Could you check a few things on this model? Use its own coordinates, in mm. Face numbers are marked on the shaded views. Coordinates: 2 decimals unless noted, no trailing zeros. Order: outer loops, then holes, each group sorted by start corner. A loop starts at its lowest first (then second) coordinate and runs counter-clockwise, first axis right, second up. Notation, with made-up numbers: (16.5, 52) -> (38.5, 52) arc R33 ccw to (38.5, 88) -> close; hole circle Ø4 at (-21.75, 65). An arc over 180 degrees is marked (long way). Use a Markdown table: item, result. Add a question column.
1) If we section it at A-A (z = 0): Write out the boundary of the cut face in (x, y).
2) If I drill on L1, parallel to X at y = 41.4, z = 0; L2, parallel to Y at x = 40, z = -10; L3, parallel to Z at x = -78.5, y = -21, over which ranges is the centre line in solid material (lowest first)? Write a range as [from, to].
3) If we section it at D-D (x = -11.5): Write out the boundary of the cut face in (y, z), plus the area to 3 significant figures.
4) Will these pins go through, and if not, where does the flat tip stop? pin 1 Ø4 at (x, y) = (-32.5, 14) entering from -Z; pin 2 Ø6 at (x, z) = (51, -12.5) entering from -Y; pin 3 Ø9 at (x, z) = (-75, 0) entering from +Y; pin 4 Ø2 at (x, z) = (-42, -4) entering from +Y.
5) If we section it at B-B (y = 0): Write out the boundary of the cut face in (x, z), plus the area to 3 significant figures.
6) Thinking about a two-plate mould opening in Y: for the marked faces 1 and 2, which applies, +Y half, -Y half, draft (parallel to the pull), parting line (faces both ways), or undercut?
Solid Edge part; units mm, degrees
sketch "Sketch1" plane through (0, 0, 0) normal (1, 0, 0) x (0, 1, 0)
  circle A0 centre (0, 0) radius 42.5
extrude "Protrusion1" add sketch "Sketch1" along normal mid plane 200
sketch "Sketch2" plane through (0, 0, 0) normal (1, 0, 0) x (0, 1, 0)
  circle A0 centre (0, 0) radius 41
extrude "ExtrudedCutout_5" cut sketch "Sketch2" along normal mid plane 200
sketch "Sketch3" plane through (0, 0, 0) normal (0, -1, 0) x (1, 0, 0)
  circle A0 centre (75, 0) radius 4
extrude "ExtrudedCutout_9" cut sketch "Sketch3" along normal mid plane 90
sketch "Sketch4" plane through (0, 0, 0) normal (0, -1, 0) x (1, 0, 0)
  circle A0 centre (-75, 0) radius 4
extrude "ExtrudedProtrusion_6" cut sketch "Sketch4" along normal mid plane 90
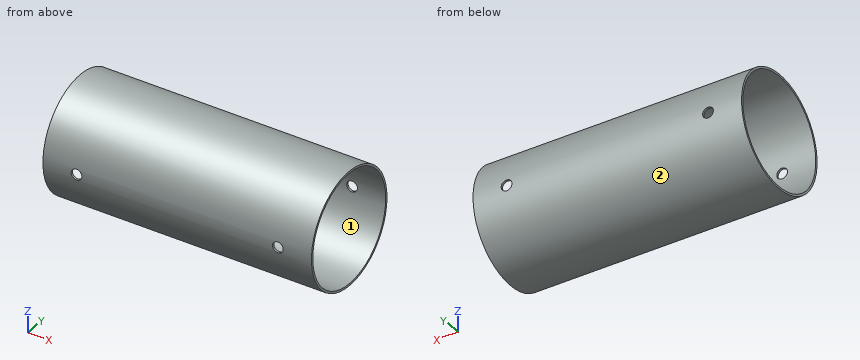
Answer sheet:
| question | item | result |
|---|---|---|
| 1 | outline | (-100, -42.5) -> (-79, -42.5) -> (-79, -41) -> (-100, -41) -> close; (-100, 41) -> (-79, 41) -> (-79, 42.5) -> (-100, 42.5) -> close; (-71, -42.5) -> (71, -42.5) -> (71, -41) -> (-71, -41) -> close; (-71, 41) -> (71, 41) -> (71, 42.5) -> (-71, 42.5) -> close; (79, -42.5) -> (100, -42.5) -> (100, -41) -> (79, -41) -> close; (79, 41) -> (100, 41) -> (100, 42.5) -> (79, 42.5) -> close |
| 2 | L1 | [-100, -79], [-71, 71], [79, 100] |
| 2 | L2 | [-41.31, -39.76], [39.76, 41.31] |
| 2 | L3 | [-36.95, -35.21], [35.21, 36.95] |
| 3 | outline | circle Ø85 at (0, 0); hole circle Ø82 at (0, 0) |
| 3 | area | 393 mm2 |
| 4 | pin 1 | z = -40.77 |
| 4 | pin 2 | y = -41.42 |
| 4 | pin 3 | y = 42.5 |
| 4 | pin 4 | y = 42.39 |
| 5 | outline | (-100, -42.5) -> (100, -42.5) -> (100, -41) -> (-100, -41) -> close; (-100, 41) -> (100, 41) -> (100, 42.5) -> (-100, 42.5) -> close |
| 5 | area | 600 mm2 |
| 6 | face 1 | undercut |
| 6 | face 2 | parting line |
